```python
from build123d import *

# Parameters (mm, degrees)
SKETCH1_RX          = 14
SKETCH1_RY          = 10
RING_EXTRUDE_DEPTH  = 1.5
SPAR_CUT_DEPTH      = 18.464249197
SPAR_CUT_DEPTH_BACK = 18.464249197


with BuildPart() as part:
    # Sketch1 → Ring extrude (new, symmetric)
    with BuildSketch(Plane.XY):
        with Locations((0, 0)):
            Ellipse(SKETCH1_RX, SKETCH1_RY)
    extrude(amount=RING_EXTRUDE_DEPTH, both=True)

    # Sketch2 → Spar cut (cut, two sides: drawn at the far end of the back side and taken through both)
    with BuildSketch(Plane.XY.offset(1.5).offset(-SPAR_CUT_DEPTH_BACK)):
        with BuildLine():
            Line((-6.35, 3.65), (-6.35, 8.912199275))
            add(Edge.make_bspline(
                [(6.35, 8.912199275), (0, 11.220574957), (-6.35, 8.912199275)],
                knots=[1.100027707, 1.100027707, 1.100027707, 2.041564947, 2.041564947, 2.041564947], degree=2, weights=[1, 0.891219928, 1]))
            Line((6.35, 8.912199275), (6.35, 3.65))
            ThreePointArc((6.35, 3.65), (0, -2.7), (-6.35, 3.65))
        make_face()
    extrude(amount=SPAR_CUT_DEPTH + SPAR_CUT_DEPTH_BACK, mode=Mode.SUBTRACT)


solid = part.part
```
For this review, take the finished solid that the model builds, in its own axes (mm). A direction names the side the tool comes from. Give positions to 0.01 mm unless a question says otherwise; leave off trailing zeros.
1) Insertion check: pin 1 (1.5 mm diameter, centred on x = -2.5, z = 0.5, fed in from +Y); pin 2 (0.9 mm diameter, centred on y = 6, z = -0.5, fed in from -X); pin 3 (0.9 mm diameter, centred on y = 6.5, z = -0.5, fed in from +X). Each pin has a flat end and moves straight along its axis. Give the tip position at first contact, or say it passes through.
2) Wall thickness on line 1 (X direction, y = 7, z = 0.05); line 2 (X direction, y = 4, z = 0.8); line 3 (Y direction, x = -2.5, z = 1.25): over which ranges is each line inside the solid? List them lowest first.
3) For faces 4 (the face through (0, -5, 1.5)), 5 (the face through (6.35, 6, 0)), list the 3-axis set-ups (+Z, -Z, +X, -X, +Y, -Y) from which the entire face can be reached by the end or side of a thin tool; tool diameter is ignored.
4) The part is to be moulded in two halves that separate along X. For faces 1 (the face through (0.1, -2.7, 0)), 2 (the face through (0, -5, -1.5)), 3 (the face through (-6.35, 6, 0)), say which applies: released by +X, released by -X, zero draft, split by the parting line, or undercut.
Derived:
1. pin 1: stops at y = -1.81
1. pin 2: stops at x = -11.65
1. pin 3: stops at x = 11.15
2. line 1: x = -10 to -6.35, 6.35 to 10
2. line 2: x = -12.83 to -6.35, 6.35 to 12.83
2. line 3: y = -9.84 to -2.19
3. face 4: +Z, +X, -X, +Y, -Y
3. face 5: +Z, -Z, +Y
4. face 1: undercut
4. face 2: zero draft
4. face 3: undercut
